Model file for the job. Use its own axes, mm. Face numbers are marked on the shaded views. A direction names the side the tool comes from. Round coordinates to 2 decimals unless told otherwise and drop trailing zeros. Order: outer loops, then holes, each group sorted by start corner. A loop starts at its lowest first (then second) coordinate and runs counter-clockwise, first axis right, second up. Notation, with made-up numbers: (-32, 2.5) - (16, 2.5) arc R22 cw to (16, 35.5) - close; hole circle Ø5 at (-8, 72). An arc over 180 degrees is marked (long way). Use one line per item in the form item = value.
from build123d import *

# Parameters (mm, degrees)
BOSS_EXTRUDE2_DEPTH = 150
SKETCH1_4_W         = 60
SKETCH1_4_H         = 60
BOSS_EXTRUDE3_DEPTH = 100
SKETCH1_5_R         = 50
SKETCH1_5_W         = 60
SKETCH1_5_H         = 60
BOSS_EXTRUDE4_DEPTH = 50


with BuildPart() as part:
    # Sketch1 → Boss-Extrude2 (new body)
    with BuildSketch(Plane.XY):
        Polygon((-22.5, -12.990381057), (22.5, -12.990381057), (0, 25.980762114), align=None)
    extrude(amount=BOSS_EXTRUDE2_DEPTH)

    # Sketch1_4 → Boss-Extrude3 (add)
    with BuildSketch(Plane.XY):
        Rectangle(SKETCH1_4_W, SKETCH1_4_H)
        Polygon((22.5, -12.990381057), (0, 25.980762114), (-22.5, -12.990381057), align=None, mode=Mode.SUBTRACT)
    extrude(amount=BOSS_EXTRUDE3_DEPTH)

    # Sketch1_5 → Boss-Extrude4 (add)
    with BuildSketch(Plane.XY):
        Circle(SKETCH1_5_R)
        Rectangle(SKETCH1_5_W, SKETCH1_5_H, mode=Mode.SUBTRACT)
    extrude(amount=BOSS_EXTRUDE4_DEPTH)


solid = part.part
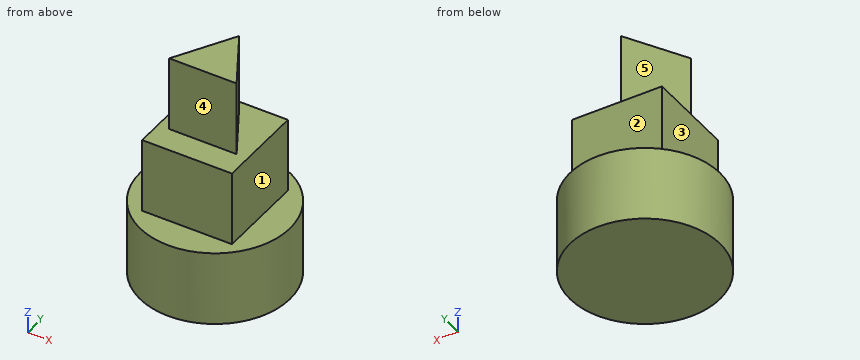
(1) Tool access for the marked faces 1, 2, 3, 4 and 5: list every direction of +Z, -Z, +X, -X, +Y, -Y with a clear straight run to the whole face (end or side of a thin tool).
Report:
face_1 = +Z, +X, +Y, -Y
face_2 = +Z, +X, -X, +Y
face_3 = +Z, -X, +Y, -Y
face_4 = +Z, +X, -X, -Y
face_5 = +Z, -X, +Y
(2) Probe probe 1 along Z at (x, y) = (-8.5, -17); probe 2 along X at (y, z) = (-11.5, 96.5); probe 3 along Z at (x, y) = (8, -38). List the from-to ranges inside material, lowest first. Write a range as [from, to].
Report:
probe_1 = [0, 100]
probe_2 = [-30, 30]
probe_3 = [0, 50]
(3) Slice it at B-B on z = 136.5. Give the cut face in (x, y).
Report:
outline = (-22.5, -12.99) - (22.5, -12.99) - (0, 25.98) - close
(4) Slice it at A-A on y = 0. Give the cut face in (x, z), then the cut area to 3 significant figures.
Report:
outline = (-50, 0) - (50, 0) - (50, 50) - (30, 50) - (30, 100) - (15, 100) - (15, 150) - (-15, 150) - (-15, 100) - (-30, 100) - (-30, 50) - (-50, 50) - close
area = 9,500 mm2
(5) Slice it at C-C on y = -23. Give the cut face in (x, z).
Report:
outline = (-44.4, 0) - (44.4, 0) - (44.4, 50) - (30, 50) - (30, 100) - (-30, 100) - (-30, 50) - (-44.4, 50) - close
(6) Slice it at D-D on z = 10.5. Give the cut face in (x, y), then the cut area to 3 significant figures.
Report:
outline = circle Ø100 at (0, 0)
area = 7,850 mm2
(7) Pin check, flat tips, straight feed: pin 1 (4 mm diameter, centred on y = -2, z = 59, fed in from +X); pin 2 (25 mm diameter, centred on x = 13, z = 64.5, fed in from +Y); pin 3 (15 mm diameter, centred on x = 0, z = 83.5, fed in from -Y). Stop position of each tip, or through.
Report:
pin_1 = 30
pin_2 = 30
pin_3 = -30
